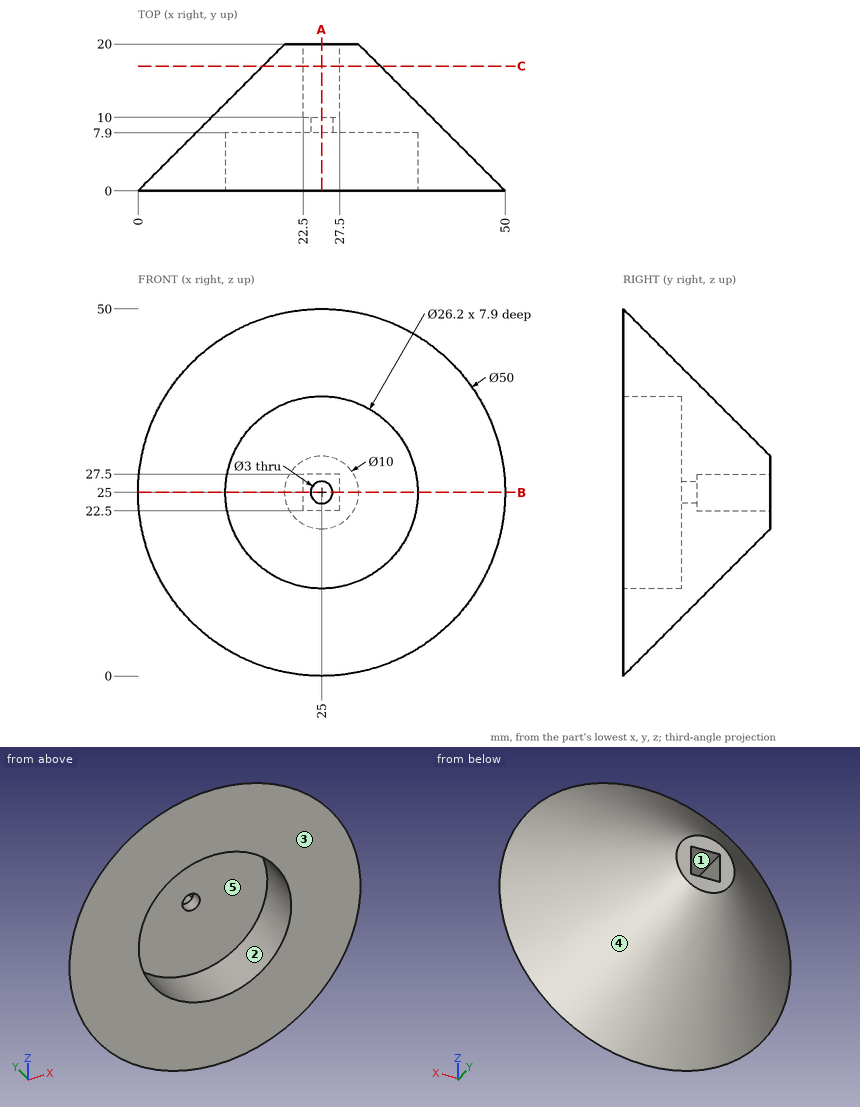
Answer from the drawing. Dimensions are ordinates in mm from the lowest x, y and z of the part. A direction names the side the tool comes from. Give positions to 0.01 mm unless a question says otherwise; leave off trailing zeros. Write each loop counter-clockwise with the first axis right and the second up, starting at its lowest first coordinate (ties: lowest second). Pieces come first, ordered by that corner, then holes.
1) For a pull along X with two mould halves and no side action, classify the marked faces 3, 4 and 5 as pulls with the +X half, pulls with the -X half, needs draft (parallel to the pull), parting line crosses it, or undercut.
2) Section B-B (z = 25) is taken. Write down the section's boundary in (x, y).
3) Find the intervals of material crossed by L1, parallel to X at y = 3.5, z = 25; L2, parallel to X at y = 5.25, z = 20.5; L3, parallel to Z at x = 34, y = 3.25, in increasing order.
4) Section C-C (y = 17) is taken. Write down the section's boundary in (x, z), and give its area (3 significant figures).
5) Section A-A (x = 25) is taken. Write down the section's boundary in (y, z).
6) A tool of negligible diameter and unlimited length cuts with its end or side. For the marked faces 1 and 2, from which of +Z, -Z, +X, -X, +Y, -Y can it reach the whole face along a straight path? Write none if from no direction.
7) Given P1, Ø4, axis at x = 39, y = 3.5, coming from the +Z side; P2, Ø2.5, axis at x = 25, y = 16.5, coming from the -Z side; P3, Ø2, axis at x = 43, y = 2, coming from the -Z side; P4, Ø2, axis at x = 43.5, y = 8, coming from the -Z side, each flat-ended and moving along its own axis, determine where each tip first touches the part or whether it passes through.
Response:
1. face 3: needs draft
1. face 4: parting line crosses it
1. face 5: undercut
2. outline: (0, 0) - (11.9, 0) - (11.9, 7.9) - (23.5, 7.9) - (23.5, 10) - (22.5, 10) - (22.5, 20) - (20, 20) - close; (26.5, 7.9) - (38.1, 7.9) - (38.1, 0) - (50, 0) - (30, 20) - (27.5, 20) - (27.5, 10) - (26.5, 10) - close
3. L1: x = 3.5 to 11.9, 38.1 to 46.5
3. L2: x = 5.77 to 12.7, 37.3 to 44.23
3. L3: z = 5.2 to 15.48, 34.52 to 44.8
4. outline: circle Ø16 at (25, 25); hole (22.5, 22.5) - (27.5, 22.5) - (27.5, 27.5) - (22.5, 27.5) - close
4. area: 176 mm2
5. outline: (0, 0) - (20, 20) - (20, 22.5) - (10, 22.5) - (10, 23.5) - (7.9, 23.5) - (7.9, 11.9) - (0, 11.9) - close; (0, 38.1) - (7.9, 38.1) - (7.9, 26.5) - (10, 26.5) - (10, 27.5) - (20, 27.5) - (20, 30) - (0, 50) - close
6. face 1: +Y
6. face 2: -Y
7. P1: stops at z = 44.25
7. P2: stops at z = 15.25
7. P3: stops at z = 8.76
7. P4: passes through
